Read the model definition and answer for the solid it produces. Units are mm, in the model's axes. A direction names the side the tool comes from. Coordinates: 2 decimals unless noted, no trailing zeros. Write each loop counter-clockwise with the first axis right and the second up, starting at its lowest first coordinate (ties: lowest second). Pieces come first, ordered by that corner, then holes.
Item 1: Section A-A (z = 44) is taken. State how many separate pieces and enclosed holes the cut face has, then the cut area to 3 significant figures.
Item 2: A tool of negligible diameter and unlimited length cuts with its end or side. For faces 4 (the face through (-5, -6, 25.4)), 5 (the face through (43, 23, -6.35)), 6 (the face through (2.48, 20.34, 30.5)), from which of +Z, -Z, +X, -X, +Y, -Y can it reach the whole face along a straight path? Write none if from no direction.
Item 3: Section D-D (x = 41) is taken. Give the vertices of the cut face in (y, z) (3 decimals).
Item 4: Each of these flat-tipped pins is pushed along its axis until it touches: P1, Ø2, axis at x = 2, z = 18, coming from the -Y side; P2, Ø10, axis at y = 29, z = -16, coming from the -X side; P3, Ø10, axis at x = 8, y = 35, coming from the -Z side. Where does it stop, or does it pass through?
Item 5: Determine the mould class of faces 1 (the face through (120.65, 2, -1)), 2 (the face through (112.824, -25.715, -39.373)), 3 (the face through (3.175, -13, 46)) for opening direction X: released by +X, released by -X, zero draft, split by the parting line, or undercut.
Item 6: Straight lines are drawn through the part: probe 1 along X at (y, z) = (-23, -42) (3 decimals); probe 2 along X at (y, z) = (0.5, 36.5); probe 3 along Y at (x, z) = (66.5, 13). For each, find the intervals that lie inside material, in ascending order.
from build123d import *

# Parameters (mm, degrees)
BOSS_EXTRUDE1_DEPTH = 53.975
SKETCH3_R           = 6.35
BOSS_EXTRUDE2_DEPTH = 133.35
SKETCH4_W           = 101.6
SKETCH4_H           = 25.718784162
CUT_EXTRUDE1_DEPTH  = 168.885161643
RIB3_REACH          = 141.447
SKETCH5_WALL_W      = 411.489550618
SKETCH5_WALL_H      = 12.7
FILLET1_R           = 3.175


with BuildPart() as part:
    # Sketch1 → Boss-Extrude1 (new, symmetric)
    with BuildSketch(Plane.XY):
        with BuildLine():
            Line((120.65, 0), (-12.7, 0))
            Line((-12.7, 0), (-12.7, 5.273793493))
            ThreePointArc((-12.7, 5.273793493), (-17.169459313, 14.945825338), (-27.432, 17.810179575))
            ThreePointArc((-27.432, 17.810179575), (-49.23989896, 23.896932331), (-58.7375, 44.45))
            Line((-58.7375, 44.45), (-46.0375, 44.45))
            ThreePointArc((-46.0375, 44.45), (-31.75, 30.1625), (-17.4625, 44.45))
            Line((-17.4625, 44.45), (-4.7625, 44.45))
            Line((-4.7625, 44.45), (-4.7625, 38.1))
            ThreePointArc((-4.7625, 38.1), (2.676987758, 20.139487758), (20.6375, 12.7))
            Line((20.6375, 12.7), (120.65, 12.7))
            Line((120.65, 12.7), (120.65, 0))
        make_face()
    extrude(amount=BOSS_EXTRUDE1_DEPTH, both=True)

    # Sketch3 → Boss-Extrude2 (add)
    with BuildSketch(Plane(origin=(120.65, 0, 0), x_dir=(0, 0, -1), z_dir=(1, 0, 0))):
        with BuildLine():
            Line((-53.975, -11.431284162), (-53.975, 0))
            Line((-53.975, 0), (-25.4, 0))
            Line((-25.4, 0), (-25.4, -11.431284162))
            ThreePointArc((-25.4, -11.431284162), (-39.6875, -25.718784162), (-53.975, -11.431284162))
        make_face()
        with Locations((-39.6875, -11.431284162)):
            Circle(SKETCH3_R, mode=Mode.SUBTRACT)
        with BuildLine():
            Line((53.975, 0), (25.4, 0))
            Line((25.4, 0), (25.4, -11.431284162))
            ThreePointArc((25.4, -11.431284162), (39.6875, -25.718784162), (53.975, -11.431284162))
            Line((53.975, -11.431284162), (53.975, 0))
        make_face()
        with Locations((39.6875, -11.431284162)):
            Circle(SKETCH3_R, mode=Mode.SUBTRACT)
    extrude(amount=-BOSS_EXTRUDE2_DEPTH)

    # Sketch4 → Cut-Extrude1 (cut, through all)
    with BuildSketch(Plane.XY.offset(53.975)):
        with Locations((53.975, -12.859392081)):
            Rectangle(SKETCH4_W, SKETCH4_H)
    extrude(amount=-CUT_EXTRUDE1_DEPTH, mode=Mode.SUBTRACT)

    # Sketch5 wall → Rib3 (add, up to next)
    with BuildSketch(Plane(origin=(56.984129031, 27.206147816, 0), x_dir=(-0.975011472973, 0.222154512832, 0), z_dir=(-0.222154512832, -0.975011472973, 0)), mode=Mode.PRIVATE) as rib3_sk1:
        Rectangle(SKETCH5_WALL_W, SKETCH5_WALL_H)
    rib3_tool1 = extrude(rib3_sk1.sketch, amount=RIB3_REACH, mode=Mode.PRIVATE) - part.part
    add(rib3_tool1.solids().sort_by_distance((56.984129031, 27.206147816, 0))[0])

    # Fillet1
    fillet1_edges = [part.edges().sort_by_distance(p)[0] for p in [
        (-4.7625, 41.275, 0),
    ]]
    fillet(fillet1_edges, radius=FILLET1_R)


solid = part.part
Established:
1. separate pieces: 3
1. enclosed holes: 0
1. area: 3,380 mm2
2. face 4: +X, -X, -Y
2. face 5: -Z, +X, +Y
2. face 6: +Z, +X, +Y
3. outline: (0, -53.975) - (12.7, -53.975) - (12.7, -6.35) - (30.848, -6.35) - (30.848, 6.35) - (12.7, 6.35) - (12.7, 53.975) - (0, 53.975) - close
4. P1: stops at y = 0
4. P2: stops at x = -56.63
4. P3: stops at z = -6.35
5. face 1: released by +X
5. face 2: zero draft
5. face 3: undercut
6. probe 1: x = -12.7 to 3.175, 104.775 to 120.65
6. probe 2: x = -12.7 to 120.65
6. probe 3: y = 0 to 12.7
